Part model, mm, in its own coordinate system. A direction names the side the tool comes from. Coordinates: 2 decimals unless noted, no trailing zeros. Order: outer loops, then holes, each group sorted by start corner. A loop starts at its lowest first (then second) coordinate and runs counter-clockwise, first axis right, second up. Notation, with made-up numbers: (87.25, 5.25) - (138.25, 5.25) arc R18 ccw to (138.25, 27.25) - close; hole circle Ø4 at (40, 43.25). An arc over 180 degrees is marked (long way). Use a Markdown table: item, result. Add a question column.
1) Saw through at D-D on x = 12.5. List the corners of the cut face in (y, z).
2) Tool access for faces 1 (the face through (12, 18, 2.31)), 2 (the face through (18.21, 11.14, -12.02)), 3 (the face through (9.782, 11.14, 3.095)), 4 (the face through (0, 1, -22)), 5 (the face through (-17.399, 10.846, 15.874)): list every direction of +Z, -Z, +X, -X, +Y, -Y with a clear straight run to the whole face (end or side of a thin tool).
3) Drop flat-ended pins along their axis: P1, Ø3.5, axis at x = 0, z = 9.01, coming from the +Y side; P2, Ø5.5, axis at x = 10.5, y = 17.5, coming from the -Z side; P3, Ø2, axis at x = 10.5, y = 8.5, coming from the -Z side; P4, Ø14.5, axis at x = -12, z = -18, coming from the +Y side. Give the stop position or say it passes through.
4) Saw through at A-A on x = 0. List the corners of the cut face in (y, z).
5) Two-plate mould, pull along Y, no slides. Class faces 6 (the face through (-9.78, 11.14, 14.92)), 7 (the face through (9, 0, -6)), 8 (the face through (11, 12, -14)): +Y half, -Y half, draft (parallel to the pull), parting line (faces both ways), or undercut.
6) Wall check: L1, parallel to Y at x = 17, z = 9; L2, parallel to X at y = 15.5, z = 13.5; L3, parallel to Y at x = 7, z = -2. Give the ranges that are in metal, low to high. Write a range as [from, to].
7) Saw through at B-B on y = 17.5. List the corners of the cut face in (x, z).
8) Saw through at C-C on x = -14. List the corners of the cut face in (y, z), then the cut area to 3 significant figures.
```python
from build123d import *

# Parameters (mm, degrees)
SKETCH1_R                = 34.445
BOSS_EXTRUDE1_DEPTH      = 22
SKETCH15_R               = 34.445
CUT_EXTRUDE2_DEPTH       = 54.450126754
CUT_EXTRUDE4_START       = -1
SKETCH17_R               = 6.2
CUT_EXTRUDE4_DEPTH       = 20
SKETCH18_R               = 7.25
CUT_EXTRUDE5_DEPTH       = 41.489614217
SKETCH19_R               = 6.25
CUT_EXTRUDE7_DEPTH       = 21
SKETCH20_R               = 9.845995641
CUT_EXTRUDE9_DEPTH       = 10
FILLET12_R               = 6
SKETCH23_R               = 4
SKETCH23_R_2             = 2
CUT_EXTRUDE10_DEPTH      = 41.489614217
CUT_EXTRUDE11_START      = -12
CUT_EXTRUDE11_DEPTH      = 29.489614217
FILLET19_R               = 3
CUT_EXTRUDE12_DEPTH      = 10
CUT_EXTRUDE12_DEPTH_BACK = 10
SKETCH25_R               = 11.1
FILLET20_R               = 2


with BuildPart() as part:
    # Sketch1 → Boss-Extrude1 (new body)
    with BuildSketch(Plane(origin=(0, 0, 0), x_dir=(1, 0, 0), z_dir=(0, 1, 0))):
        with Locations(Location((0, 0, 0), (0, 0, 270))):
            Circle(SKETCH1_R)
    extrude(amount=BOSS_EXTRUDE1_DEPTH)

    # Sketch15 → Cut-Extrude2 (cut, through all)
    with BuildSketch(Plane(origin=(0, 22, 0), x_dir=(1, 0, 0), z_dir=(0, 1, 0))):
        Circle(SKETCH15_R)
        with BuildLine():
            Line((-19.109582045, 20.616901016), (-19.109582045, -17.678671312))
            Line((-19.109582045, -17.678671312), (19.109582045, -17.678671312))
            Line((19.109582045, -17.678671312), (19.109582045, 20.616901016))
            ThreePointArc((19.109582045, 20.616901016), (0, 28.111078483), (-19.109582045, 20.616901016))
        make_face(mode=Mode.SUBTRACT)
    extrude(amount=-CUT_EXTRUDE2_DEPTH, mode=Mode.SUBTRACT)

    # Sketch17 → Cut-Extrude4 (cut)
    with BuildSketch(Plane(origin=(0, 22, 0), x_dir=(1, 0, 0), z_dir=(0, 1, 0)).offset(CUT_EXTRUDE4_START)):
        with Locations(Location((-11.644122412, -9.008465082, 0), (0, 0, 270))):
            Circle(SKETCH17_R)
        with Locations(Location((11.644122412, -9.008465082, 0), (0, 0, 90))):
            Circle(SKETCH17_R)
    extrude(amount=-CUT_EXTRUDE4_DEPTH, mode=Mode.SUBTRACT)

    # Sketch18 → Cut-Extrude5 (cut, through all)
    with BuildSketch(Plane(origin=(0, 22, 0), x_dir=(1, 0, 0), z_dir=(0, 1, 0))):
        with Locations(Location((0, 5.846291401, 0), (0, 0, 270))):
            Circle(SKETCH18_R)
    extrude(amount=-CUT_EXTRUDE5_DEPTH, mode=Mode.SUBTRACT)

    # Sketch19 → Cut-Extrude7 (cut)
    with BuildSketch(Plane(origin=(0, 22, 0), x_dir=(1, 0, 0), z_dir=(0, 1, 0))):
        with Locations((0, 22.497935332)):
            Circle(SKETCH19_R)
    extrude(amount=-CUT_EXTRUDE7_DEPTH, mode=Mode.SUBTRACT)

    # Sketch20 → Cut-Extrude9 (cut)
    with BuildSketch(Plane(origin=(0, 22, 0), x_dir=(1, 0, 0), z_dir=(0, 1, 0))):
        with Locations(Location((0, 5.846291401, 0), (0, 0, 270))):
            Circle(SKETCH20_R)
    extrude(amount=-CUT_EXTRUDE9_DEPTH, mode=Mode.SUBTRACT)

    # Fillet12
    fillet12_edges = [part.edges().sort_by_distance(p)[0] for p in [
        (-19.109582045, 11, 17.678671312),
        (19.109582045, 11, 17.678671312),
    ]]
    fillet(fillet12_edges, radius=FILLET12_R)

    # Sketch23 → Cut-Extrude10 (cut, through all)
    with BuildSketch(Plane(origin=(0, 22, 0), x_dir=(1, 0, 0), z_dir=(0, 1, 0))):
        with Locations(Location((-11.644122412, -9.008465082, 0), (0, 0, 270))):
            Circle(SKETCH23_R)
        with Locations(Location((11.644122412, -9.008465082, 0), (0, 0, 270))):
            Circle(SKETCH23_R)
        with Locations(Location((0, -9.008465082, 0), (0, 0, 270))):
            Circle(SKETCH23_R_2)
    extrude(amount=-CUT_EXTRUDE10_DEPTH, mode=Mode.SUBTRACT)

    # Sketch24 → Cut-Extrude11 (cut, through all)
    with BuildSketch(Plane.XZ.offset(CUT_EXTRUDE11_START)):
        with BuildLine():
            Line((-19.109582045, -20.616901016), (-19.109582045, 2.30978602))
            Line((-19.109582045, 2.30978602), (19.109582045, 2.30978602))
            Line((19.109582045, 2.30978602), (19.109582045, -20.616901016))
            ThreePointArc((19.109582045, -20.616901016), (0, -28.111078483), (-19.109582045, -20.616901016))
        make_face()
    extrude(amount=-CUT_EXTRUDE11_DEPTH, mode=Mode.SUBTRACT)

    # Fillet19
    fillet19_edges = [part.edges().sort_by_distance(p)[0] for p in [
        (-19.109582045, 17, 2.30978602),
        (12.31259954, 12, 2.30978602),
        (-12.31259954, 12, 2.30978602),
        (-19.109582045, 12, -9.153557498),
        (19.109582045, 12, -9.153557498),
        (19.109582045, 17, 2.30978602),
    ]]
    fillet(fillet19_edges, radius=FILLET19_R)

    # Sketch25 → Cut-Extrude12 (cut, two sides: drawn at the far end of the back side and taken through both)
    with BuildSketch(Plane(origin=(0, 12, 0), x_dir=(1, 0, 0), z_dir=(0, 1, 0)).offset(-CUT_EXTRUDE12_DEPTH_BACK)):
        with Locations((0, 5.846291401)):
            Circle(SKETCH25_R)
    extrude(amount=CUT_EXTRUDE12_DEPTH + CUT_EXTRUDE12_DEPTH_BACK, mode=Mode.SUBTRACT)

    # Fillet20
    fillet20_edges = [part.edges().sort_by_distance(p)[0] for p in [
        (-2.330818134, 7, -16.698815845),
        (2.330818134, 7, -16.698815845),
    ]]
    fillet(fillet20_edges, radius=FILLET20_R)


solid = part.part
```
Results are:
| question | item | result |
|---|---|---|
| 1 | outline | (0, -25.18) - (12, -25.18) - (12, -0.69) arc R3 cw to (15, 2.31) - (22, 2.31) - (22, 5.1) - (21, 5.1) - (21, 2.87) - (1, 2.87) - (1, 5.1) - (0, 5.1) - close; (0, 12.92) - (1, 12.92) - (1, 15.15) - (21, 15.15) - (21, 12.92) - (22, 12.92) - (22, 17.68) - (0, 17.68) - close |
| 2 | face 1 | -Z, +X, -X, +Y |
| 2 | face 2 | -Z, +X, +Y |
| 2 | face 3 | none |
| 2 | face 4 | +Y |
| 2 | face 5 | +Z, -X, +Y, -Y |
| 3 | P1 | through |
| 3 | P2 | z = 2.3 |
| 3 | P3 | z = -26.46 |
| 3 | P4 | y = 12 |
| 4 | outline | (0, -28.11) - (1, -28.11) - (1, -16.25) - (2, -16.25) - (2, -13.1) - (0, -13.1) - close; (0, 1.4) - (2, 1.4) - (2, 5.25) - (22, 5.25) - (22, 7.01) - (0, 7.01) - close; (0, 11.01) - (22, 11.01) - (22, 17.68) - (0, 17.68) - close |
| 5 | face 6 | undercut |
| 5 | face 7 | -Y half |
| 5 | face 8 | +Y half |
| 6 | L1 | [0, 1], [21, 22] |
| 6 | L2 | [-18.83, -15.92], [-7.37, 7.37], [15.92, 18.83] |
| 6 | L3 | [0, 2] |
| 7 | outline | (-19.11, 5.31) arc R3 ccw to (-16.11, 2.31) - (-7.53, 2.31) arc R11.1 cw to (7.53, 2.31) - (16.11, 2.31) arc R3 ccw to (19.11, 5.31) - (19.11, 11.68) arc R6 ccw to (13.11, 17.68) - (-13.11, 17.68) arc R6 ccw to (-19.11, 11.68) - close; hole circle Ø12.4 at (-11.64, 9.01); hole circle Ø4 at (0, 9.01); hole circle Ø12.4 at (11.64, 9.01) |
| 8 | outline | (0, -24.38) - (12, -24.38) - (12, -0.69) arc R3 cw to (15, 2.31) - (22, 2.31) - (22, 5.78) - (21, 5.78) - (21, 3.27) - (1, 3.27) - (1, 5.78) - (0, 5.78) - close; (0, 12.24) - (1, 12.24) - (1, 14.74) - (21, 14.74) - (21, 12.24) - (22, 12.24) - (22, 17.61) - (0, 17.61) - close |
| 8 | area | 416 mm2 |
